Source: CAD feature listing. Evaluate the final solid. Frame: model axes, mm. Face numbers are marked on the shaded views. Round coordinates to 2 decimals unless told otherwise and drop trailing zeros. Loops run counter-clockwise (first coordinate to the right, second up) from the corner with the lowest first, then second, coordinate; pieces in that order, holes last.
(1) First-contact query: pin 1 Ø3 at (x, z) = (-8, 0) entering from +Y; pin 2 Ø1 at (y, z) = (4, -20) entering from +X; pin 3 Ø8 at (x, z) = (7, -5) entering from -Y; pin 4 Ø1 at (x, y) = (-10, 3) entering from +Z. Flat tips, straight axial feed; report the tip coordinate or a pass-through.
(2) Section A-A, the plane x = 1. Return the cut outline in (y, z), plus the area to 3 significant figures.
(3) Section C-C, the plane x = -8. Return the cut outline in (y, z).
(4) Section B-B, the plane z = -7.5. Return the cut outline in (x, y), plus the area to 3 significant figures.
(5) Mould query, pull axis X, two halves, no side actions, for the marked faces 1, 2 and 3. Classes: pulls with the +X half, pulls with the -X half, needs draft (parallel to the pull), parting line crosses it, or undercut.
(6) Material intervals for probe 1 along X at (y, z) = (4.1, 0); probe 2 along X at (y, z) = (3.3, -10); probe 3 along X at (y, z) = (2.95, 8.5), sorted ascending.
(7) Section D-D, the plane z = 24. Return the cut outline in (x, y), plus the area to 3 significant figures.
```python
from build123d import *

# Parameters (mm, degrees)
SKETCH1_R           = 28.5
SKETCH1_R_2         = 2.5
BOSS_EXTRUDE1_DEPTH = 6
CUT_EXTRUDE1_DEPTH  = 8
SKETCH3_R           = 1.8
CUT_EXTRUDE2_DEPTH  = 10.54


with BuildPart() as part:
    # Sketch1 → Boss-Extrude1 (new body)
    with BuildSketch(Plane(origin=(0, 0, 0), x_dir=(1, 0, 0), z_dir=(0, 1, 0))):
        with Locations(Location((0, 0, 0), (0, 0, 270))):
            Circle(SKETCH1_R)
        with Locations(Location((0, 23.5, 0), (0, 0, 270))):
            Circle(SKETCH1_R_2, mode=Mode.SUBTRACT)
        with Locations(Location((20.351596989, 11.75, 0), (0, 0, 270))):
            Circle(SKETCH1_R_2, mode=Mode.SUBTRACT)
        with Locations(Location((20.351596989, -11.75, 0), (0, 0, 270))):
            Circle(SKETCH1_R_2, mode=Mode.SUBTRACT)
        with Locations(Location((0, -23.5, 0), (0, 0, 270))):
            Circle(SKETCH1_R_2, mode=Mode.SUBTRACT)
        with Locations(Location((-20.351596989, -11.75, 0), (0, 0, 270))):
            Circle(SKETCH1_R_2, mode=Mode.SUBTRACT)
        with Locations(Location((-20.351596989, 11.75, 0), (0, 0, 270))):
            Circle(SKETCH1_R_2, mode=Mode.SUBTRACT)
    extrude(amount=BOSS_EXTRUDE1_DEPTH)

    # Sketch2 → Cut-Extrude1 (cut)
    with BuildSketch(Plane(origin=(0, 6, 0), x_dir=(1, 0, 0), z_dir=(0, 1, 0))):
        Polygon((-0.284546252, -2.872693294), (2.345552244, -1.68277093), (2.630098496, 1.189922365), (0.284546252, 2.872693294), (-2.345552244, 1.68277093), (-2.630098496, -1.189922365), align=None)
    extrude(amount=-CUT_EXTRUDE1_DEPTH, mode=Mode.SUBTRACT)

    # Sketch3 → Cut-Extrude2 (cut)
    with BuildSketch(Plane(origin=(0, 6, 0), x_dir=(1, 0, 0), z_dir=(0, 1, 0))):
        with Locations(Location((8, 0, 0), (0, 0, 270))):
            Circle(SKETCH3_R)
        with Locations(Location((4, -6.92820323, 0), (0, 0, 270))):
            Circle(SKETCH3_R)
        with Locations(Location((-4, -6.92820323, 0), (0, 0, 270))):
            Circle(SKETCH3_R)
        with Locations(Location((-8, 0, 0), (0, 0, 270))):
            Circle(SKETCH3_R)
        with Locations(Location((-4, 6.92820323, 0), (0, 0, 270))):
            Circle(SKETCH3_R)
        with Locations(Location((4, 6.92820323, 0), (0, 0, 270))):
            Circle(SKETCH3_R)
    extrude(amount=-CUT_EXTRUDE2_DEPTH, mode=Mode.SUBTRACT)


solid = part.part
```
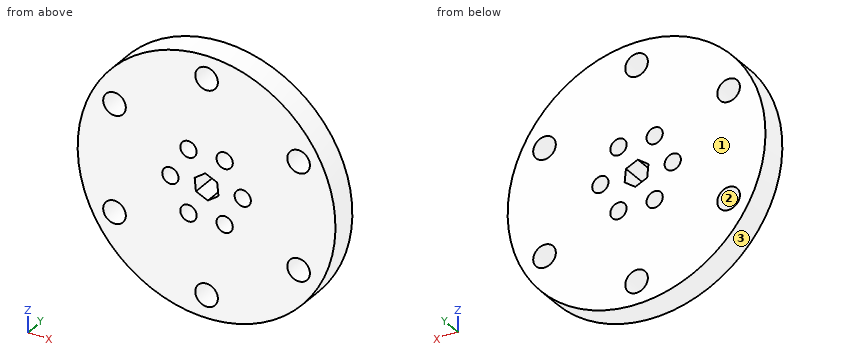
Output values:
1. pin 1: passes through
1. pin 2: stops at x = 20.78
1. pin 3: stops at y = 0
1. pin 4: stops at z = 26.87
2. outline: (0, -28.48) - (6, -28.48) - (6, -25.79) - (0, -25.79) - close; (0, -21.21) - (6, -21.21) - (6, -2.36) - (0, -2.36) - close; (0, 2.29) - (6, 2.29) - (6, 21.21) - (0, 21.21) - close; (0, 25.79) - (6, 25.79) - (6, 28.48) - (0, 28.48) - close
2. area: 259 mm2
3. outline: (0, -27.35) - (6, -27.35) - (6, -1.8) - (0, -1.8) - close; (0, 1.8) - (6, 1.8) - (6, 27.35) - (0, 27.35) - close
4. outline: (-27.5, 0) - (-5.71, 0) - (-5.71, 6) - (-27.5, 6) - close; (-2.29, 0) - (2.29, 0) - (2.29, 6) - (-2.29, 6) - close; (5.71, 0) - (27.5, 0) - (27.5, 6) - (5.71, 6) - close
4. area: 289 mm2
5. face 1: needs draft
5. face 2: undercut
5. face 3: parting line crosses it
6. probe 1: x = -28.5 to -9.8, -6.2 to -2.51, 2.51 to 6.2, 9.8 to 28.5
6. probe 2: x = -26.69 to -22.14, -18.57 to 18.57, 22.14 to 26.69
6. probe 3: x = -27.2 to -4.88, -3.12 to 3.12, 4.88 to 27.2
7. outline: (-15.37, 0) - (-2.45, 0) - (-2.45, 6) - (-15.37, 6) - close; (2.45, 0) - (15.37, 0) - (15.37, 6) - (2.45, 6) - close
7. area: 155 mm2
